For this review, take the finished solid that the model builds, in its own axes (mm). A direction names the side the tool comes from. Round coordinates to 2 decimals unless told otherwise and drop trailing zeros. Write each loop counter-clockwise with the first axis right and the second up, starting at its lowest first coordinate (ties: lowest second). Pieces come first, ordered by that corner, then holes. Notation, with made-up numbers: (-25, 78) -> (-11, 78) arc R27 cw to (-11, 110) -> close; hole circle Ø2 at (45.25, -10.5). An arc over 180 degrees is marked (long way). Write each question's results on one line, items separated by ' | '. Start each with the question number.
Item 1: To check wall thickness, follow line 1 along X through (y, z) = (27.75, -17); line 2 along Z through (x, y) = (7, 15.25); line 3 along X through (y, z) = (5.25, -17). State the ranges of each line that lie inside material, in increasing order.
Item 2: Clearance check with flat-ended pins moving along their axes: pin 1 (10 mm diameter, centred on x = -4, y = 3, fed in from +Z); pin 2 (6 mm diameter, centred on x = 7, z = -17, fed in from +Y). State where each tip first meets the part, or that it passes through.
Item 3: Add section D-D (x = 10). State the section outline as (y, z) points, plus the area to 3 significant figures.
Item 4: The part is to be moulded in two halves that separate along Y. For faces 1 (the flat face through (0, 25, -10)), 2 (the flat face through (0, 30, -13)), 3 (the flat face through (-14.79, 21.71, -1)), 4 (the flat face through (0, 15, -24.8)), say which applies: +Y half, -Y half, draft (parallel to the pull), parting line (faces both ways), or undercut.
Item 5: Add section C-C (z = -20). State the section outline as (x, y) points, plus the area to 3 significant figures.
Item 6: Add section A-A (z = -17). State the section outline as (x, y) points.
Item 7: Add section B-B (y = 11.25). State the section outline as (x, z) points.
Item 8: Tool access review of faces 5 (the flat face through (-15, 23, -17.5)), 6 (the cylindrical face through (14.51, 21.71, -5.88)), 7 (the flat face through (0, 15, 0)), 8 (the flat face through (14.78, 21.71, -1.03)): name each direction out of +Z, -Z, +X, -X, +Y, -Y from which nothing blocks a thin tool from reaching the whole face with its end or side.
from build123d import *
from OCP.BRepFilletAPI import BRepFilletAPI_MakeChamfer

# Parameters (mm, degrees)
BOSS_EXTRUDE1_DEPTH             = 30
CUT_EXTRUDE2_DEPTH              = 5.5
CBORE_FOR_M4_SBHCS1_D           = 4.5
CBORE_FOR_M4_SBHCS1_CBORE_D     = 8.6
CBORE_FOR_M4_SBHCS1_CBORE_DEPTH = 8
F_3_9_3_9_DIAMETER_HOLE1_D      = 3.9
CUT_EXTRUDE3_DEPTH              = 43.884029661
CUT_EXTRUDE3_DEPTH_BACK         = 43.884029661
SKETCH9_W                       = 7.5
SKETCH9_H                       = 8
CHAMFER1_SIZE                   = 4
CHAMFER1_SIZE2                  = 3.37362922
DELETEFACE1_START               = 24.5
DELETEFACE1_DEPTH               = 2.5
DELETEFACE2_START               = 19
DELETEFACE2_DEPTH               = 5.5
FILLET1_R                       = 10


# Read off the part's stored shape, not the designer's step: DeleteFace1, DeleteFace2
with BuildPart() as part:
    # Sketch1 → Boss-Extrude1 (new body)
    with BuildSketch(Plane(origin=(0, 0, 0), x_dir=(1, 0, 0), z_dir=(0, 1, 0))):
        Polygon((-18, 0), (18, 0), (18, 20.8), (14, 24.8), (-14, 24.8), (-18, 20.8), align=None)
    extrude(amount=BOSS_EXTRUDE1_DEPTH)

    # Sketch7 → Cut-Extrude2 (cut)
    with BuildSketch(Plane(origin=(0, 19, 0), x_dir=(1, 0, 0), z_dir=(0, 1, 0))):
        with BuildLine():
            Line((-7, 21.3), (7, 21.3))
            ThreePointArc((7, 21.3), (9.706928791, 20.34103824), (11.206489583, 17.891877451))
            Line((11.206489583, 17.891877451), (15, 0))
            Line((15, 0), (-15, 0))
            Line((-15, 0), (-11.206489583, 17.891877451))
            ThreePointArc((-11.206489583, 17.891877451), (-9.706928791, 20.34103824), (-7, 21.3))
        make_face()
    extrude(amount=CUT_EXTRUDE2_DEPTH, mode=Mode.SUBTRACT)

    # CBORE for M4 SBHCS1 (through all)
    with Locations(Plane(origin=(0, 30, 0), x_dir=(1, 0, 0), z_dir=(0, 1, 0))):
        with Locations((-7, 17), (7, 17)):
            CounterBoreHole(CBORE_FOR_M4_SBHCS1_D / 2, CBORE_FOR_M4_SBHCS1_CBORE_D / 2, CBORE_FOR_M4_SBHCS1_CBORE_DEPTH)

    # Ø3.9 (3.9) Diameter Hole1 (through all)
    with Locations(Plane(origin=(0, 30, 0), x_dir=(1, 0, 0), z_dir=(0, 1, 0))):
        with Locations((-7, 6), (7, 6)):
            Hole(F_3_9_3_9_DIAMETER_HOLE1_D / 2)

    # Sketch9 → Cut-Extrude3 (cut, two sides: drawn at the far end of the back side and taken through both)
    with BuildSketch(Plane(origin=(0, 0, 0), x_dir=(0, 0, -1), z_dir=(1, 0, 0)).offset(-CUT_EXTRUDE3_DEPTH_BACK)):
        with Locations((13.75, 23)):
            Rectangle(SKETCH9_W, SKETCH9_H)
    extrude(amount=CUT_EXTRUDE3_DEPTH + CUT_EXTRUDE3_DEPTH_BACK, mode=Mode.SUBTRACT)

    # Chamfer1: one chamfer whose edges measure the first distance from different faces: ONE call of the kernel's chamfer builder (chamfer() names one face for all edges)
    chamfer1_edges_1 = [part.edges().sort_by_distance(p)[0] for p in [
        (-12.879758328, 21.75, -10),
    ]]
    chamfer1_side_1 = [part.faces().sort_by_distance(p)[0] for p in [
        (-13.939879164, 21.75, -5),
    ]]
    chamfer1_edges_2 = [part.edges().sort_by_distance(p)[0] for p in [
        (12.879758328, 21.75, -10),
    ]]
    chamfer1_side_2 = [part.faces().sort_by_distance(p)[0] for p in [
        (13.939879164, 21.75, -5),
    ]]
    chamfer1 = BRepFilletAPI_MakeChamfer(part.part.solid().wrapped)
    for e in chamfer1_edges_1:
        chamfer1.Add(CHAMFER1_SIZE, CHAMFER1_SIZE2, e.wrapped, chamfer1_side_1[0].wrapped)  # the first distance lies on this face
    for e in chamfer1_edges_2:
        chamfer1.Add(CHAMFER1_SIZE, CHAMFER1_SIZE2, e.wrapped, chamfer1_side_2[0].wrapped)  # the first distance lies on this face
    add(Compound.cast(chamfer1.Shape()), mode=Mode.REPLACE)

    # DeleteFace1 outline → DeleteFace1 (cut)
    with BuildSketch(Plane(origin=(0, 0, 0), x_dir=(1, 0, 0), z_dir=(0, 1, 0)).offset(DELETEFACE1_START)):
        with BuildLine():
            Line((7, 21.3), (-7, 21.3))
            ThreePointArc((-7, 21.3), (-4.141678814, 20.212475681), (-2.729168699, 17.5))
            Line((-2.729168699, 17.5), (2.729168699, 17.5))
            ThreePointArc((2.729168699, 17.5), (4.141678814, 20.212475681), (7, 21.3))
        make_face()
    extrude(amount=DELETEFACE1_DEPTH, mode=Mode.SUBTRACT)

    # DeleteFace2 outline → DeleteFace2 (add)
    with BuildSketch(Plane(origin=(0, 0, 0), x_dir=(1, 0, 0), z_dir=(0, 1, 0)).offset(DELETEFACE2_START)):
        with BuildLine():
            Line((-11.206489583, 17.891877451), (-11.289577073, 17.5))
            Line((-11.289577073, 17.5), (-11.270831301, 17.5))
            ThreePointArc((-11.270831301, 17.5), (-11.243186813, 17.696681903), (-11.206489583, 17.891877451))
        make_face()
        with BuildLine():
            Line((11.289577073, 17.5), (11.206489583, 17.891877451))
            ThreePointArc((11.206489583, 17.891877451), (11.243186813, 17.696681903), (11.270831301, 17.5))
            Line((11.270831301, 17.5), (11.289577073, 17.5))
        make_face()
    extrude(amount=DELETEFACE2_DEPTH)

    # Fillet1
    fillet1_edges = [part.edges().sort_by_distance(p)[0] for p in [
        (-13.70941177, 21.75, -6.086986434),
        (13.70941177, 21.75, -6.086986434),
    ]]
    fillet(fillet1_edges, radius=FILLET1_R)


solid = part.part
Responses:
1) line 1: x = -18 to -11.3, -2.7 to 2.7, 11.3 to 18 | line 2: z = -24.8 to -19.25, -14.75 to -7.95, -4.05 to 0 | line 3: x = -18 to -9.25, -4.75 to 4.75, 9.25 to 18
2) pin 1: stops at z = 0 | pin 2: stops at y = 19
3) outline: (0, -24.8) -> (30, -24.8) -> (30, -20.08) -> (19, -20.08) -> (19, 0) -> (0, 0) -> close; (24.5, -10) -> (27, -10) -> (27, -13.92) -> (30, -13.92) -> (30, 0) -> (24.5, 0) -> close | area: 590 mm^2
4) face 1: undercut | face 2: +Y half | face 3: undercut | face 4: draft
5) outline: (-18, 0) -> (18, 0) -> (18, 30) -> (10.08, 30) -> (10.08, 19) -> (-10.08, 19) -> (-10.08, 30) -> (-18, 30) -> close; (-3.92, 27) -> (3.92, 27) -> (3.92, 30) -> (-3.92, 30) -> close | area: 882 mm^2
6) outline: (-18, 0) -> (-9.25, 0) -> (-9.25, 19) -> (-18, 19) -> close; (-18, 27) -> (-11.3, 27) -> (-11.3, 30) -> (-18, 30) -> close; (-4.75, 0) -> (4.75, 0) -> (4.75, 19) -> (-4.75, 19) -> close; (-2.7, 27) -> (2.7, 27) -> (2.7, 30) -> (-2.7, 30) -> close; (9.25, 0) -> (18, 0) -> (18, 19) -> (9.25, 19) -> close; (11.3, 27) -> (18, 27) -> (18, 30) -> (11.3, 30) -> close
7) outline: (-18, -20.8) -> (-14, -24.8) -> (14, -24.8) -> (18, -20.8) -> (18, 0) -> (-18, 0) -> close; hole circle Ø4.5 at (-7, -17); hole circle Ø3.9 at (-7, -6); hole circle Ø4.5 at (7, -17); hole circle Ø3.9 at (7, -6)
8) face 5: +X, -X | face 6: none | face 7: +Z, +X, -X, +Y, -Y | face 8: +Z
